Read the model definition and answer for the solid it produces. Units are mm, in the model's axes. A direction names the side the tool comes from. Round coordinates to 2 decimals unless told otherwise and drop trailing zeros. Write each loop counter-clockwise with the first axis right and the second up, starting at its lowest first coordinate (ties: lowest second). Pieces come first, ordered by that corner, then holes. Notation, with made-up numbers: (35.25, -14) - (61.25, -14) arc R16 cw to (61.25, 15) - close; hole circle Ø3 at (-33, 4.5). An arc over 180 degrees is marked (long way). One line per item, written item: value. Start each with the question number.
(1) A cutting plane is placed at D-D, the plane z = 36. Determine the outline of the cut face in (x, y), plus the area to 3 significant figures.
(2) Flat-ended cylindrical pins translate along their axes: pin 1 Ø2 at (x, y) = (7, -5) entering from -Z; pin 2 Ø3.5 at (x, z) = (15, 26) entering from -Y; pin 3 Ø8 at (x, z) = (22.5, 16) entering from -Y. Find the tip coordinate at first contact, or state that the pin passes through.
(3) A cutting plane is placed at A-A, the plane y = -12.25. Determine the outline of the cut face in (x, z), plus the area to 3 significant figures.
(4) The mould has two halves that part along X. Classify faces 1 (the face through (15, 0, 20)), 2 (the face through (12.34, -7.29, 12.68)), 3 (the face through (0, -9, 20)): +X half, -X half, draft (parallel to the pull), parting line (faces both ways), or undercut.
(5) A cutting plane is placed at C-C, the plane x = 3. Determine the outline of the cut face in (y, z), plus the area to 3 significant figures.
(6) A cutting plane is placed at B-B, the plane z = 31. Determine the outline of the cut face in (x, y), plus the area to 3 significant figures.
(7) For faces 4 (the face through (19.988, -13.435, 0.986)), 5 (the face through (15, -7, 40)), 6 (the face through (21.338, -0.435, 12.208)), 7 (the face through (15, -10, 20)), 8 (the face through (30, -9, 20)), determine the directions among +Z, -Z, +X, -X, +Y, -Y from which every point of the face is accessible in a straight line to the end or side of a thin tool.
(8) Find the intervals of material crossed by L1, parallel to X at y = -11, z = 16; L2, parallel to Z at x = 25.25, y = -12; L3, parallel to X at y = -7.25, z = 4, in increasing order.
from build123d import *

# Parameters (mm, degrees)
SKETCH_1_W          = 30
SKETCH_1_H          = 14
EXTRUDE_1_DEPTH     = 40
CUT_EXTRUDE_1_DEPTH = 35
SKETCH_4_W          = 27
SKETCH_4_H          = 36
CUT_EXTRUDE_2_DEPTH = 7.21308
SKETCH_5_R          = 0.565
CUT_EXTRUDE_3_DEPTH = 10
EXTRUDE_2_REACH     = 53.923
SKETCH_6_R          = 0.565
CUT_EXTRUDE_4_DEPTH = 1
SKETCH_8_R          = 0.565
CUT_EXTRUDE_5_DEPTH = 51.1269475


with BuildPart() as part:
    # 草图1 → 凸台-拉伸1 (new body)
    with BuildSketch(Plane.XY):
        with Locations((15, -7)):
            Rectangle(SKETCH_1_W, SKETCH_1_H)
    extrude(amount=EXTRUDE_1_DEPTH)

    # 草图3 → 切除-拉伸1 (cut)
    with BuildSketch(Plane(origin=(0, 0, 0), x_dir=(-1, 0, 0), z_dir=(0, 0, -1))):
        Polygon((-30, -4.5), (-25.764705882, -11.286920048), (-18.553603331, -6.786920048), (-22.788897449, 0), (-30, 0), align=None)
        Polygon((-7.211102551, 0), (-11.446396669, -6.786920048), (-4.235294118, -11.286920048), (0, -4.5), (0, 0), align=None)
    extrude(amount=-CUT_EXTRUDE_1_DEPTH, mode=Mode.SUBTRACT)

    # 草图4 → 切除-拉伸2 (cut)
    with BuildSketch(Plane.XZ.offset(14)):
        with Locations((15, 20)):
            Rectangle(SKETCH_4_W, SKETCH_4_H)
    extrude(amount=-CUT_EXTRUDE_2_DEPTH, mode=Mode.SUBTRACT)

    # 草图5 → 切除-拉伸3 (cut)
    with BuildSketch(Plane(origin=(0, 0, 0), x_dir=(-1, 0, 0), z_dir=(0, 0, -1))):
        with Locations((-10, -14)):
            Circle(SKETCH_5_R)
        with Locations((-20, -14)):
            Circle(SKETCH_5_R)
    extrude(amount=-CUT_EXTRUDE_3_DEPTH, mode=Mode.SUBTRACT)

    # 草图7 → 凸台-拉伸2 (add, up to next)
    with BuildSketch(Plane(origin=(0, 0, 0), x_dir=(-1, 0, 0), z_dir=(0, 0, -1)), mode=Mode.PRIVATE) as extrude_2_sk1:
        Polygon((-22.788897449, 0), (-18.553603331, -6.786920048), (-16.548520242, -10), (-13.451479758, -10), (-11.446396669, -6.786920048), (-7.211102551, 0), align=None)
    extrude_2_tool1 = extrude(extrude_2_sk1.sketch, amount=-EXTRUDE_2_REACH, mode=Mode.PRIVATE) - part.part
    add(extrude_2_tool1.solids().sort_by_distance((15, -3.886134, 0))[0])

    # 草图6 → 切除-拉伸4 (cut)
    with BuildSketch(Plane(origin=(5.189997684, 3.238754325, 0), x_dir=(0, 0, 1), z_dir=(-0.8483650059915271, -0.5294117647058821, 0))):
        with Locations(Location((12.2, -12.417642527, 0), (0, 0, 270))):
            Circle(SKETCH_6_R)
        with Locations(Location((12.2, -4.917642527, 0), (0, 0, 270))):
            Circle(SKETCH_6_R)
        with Locations(Location((4.2, -4.917642527, 0), (0, 0, 270))):
            Circle(SKETCH_6_R)
        with Locations(Location((19.97, -4.917642527, 0), (0, 0, 270))):
            Circle(SKETCH_6_R)
        with Locations(Location((27.74, -4.917642527, 0), (0, 0, 270))):
            Circle(SKETCH_6_R)
    cut_extrude_4 = extrude(amount=-CUT_EXTRUDE_4_DEPTH, mode=Mode.SUBTRACT)

    # 镜向1: 切除-拉伸4 across plane
    add(cut_extrude_4.mirror(Plane(origin=(15, 0, 0), x_dir=(0, 0, 1), z_dir=(1, 0, 0))), mode=Mode.SUBTRACT)

    # 草图8 → 切除-拉伸5 (cut, through all)
    with BuildSketch(Plane(origin=(5.189997684, 3.238754325, 0), x_dir=(0, 0, 1), z_dir=(-0.8483650059915271, -0.5294117647058821, 0))):
        with Locations(Location((12.2, -12.417642527, 0), (0, 0, 270))):
            Circle(SKETCH_8_R)
        with Locations(Location((4.2, -4.917642527, 0), (0, 0, 270))):
            Circle(SKETCH_8_R)
        with Locations(Location((27.74, -4.917642527, 0), (0, 0, 270))):
            Circle(SKETCH_8_R)
        with Locations(Location((19.97, -4.917642527, 0), (0, 0, 270))):
            Circle(SKETCH_8_R)
        with Locations(Location((12.2, -4.917642527, 0), (0, 0, 270))):
            Circle(SKETCH_8_R)
    extrude(amount=CUT_EXTRUDE_5_DEPTH, mode=Mode.SUBTRACT)


solid = part.part
Here are the results:
1. outline: (0, -14) - (1.5, -14) - (1.5, -6.79) - (11.45, -6.79) - (13.45, -10) - (16.55, -10) - (18.55, -6.79) - (28.5, -6.79) - (28.5, -14) - (30, -14) - (30, 0) - (0, 0) - close
1. area: 242 mm²
2. pin 1: z = 35
2. pin 2: y = -10
2. pin 3: y = -6.87
3. outline: (0, 0) - (30, 0) - (30, 40) - (0, 40) - close; hole (1.5, 2) - (28.5, 2) - (28.5, 38) - (1.5, 38) - close
3. area: 228 mm²
4. face 1: draft
4. face 2: undercut
4. face 3: -X half
5. outline: (-14, 0) - (-9.31, 0) - (-9.31, 2) - (-14, 2) - close; (-14, 38) - (-6.79, 38) - (-6.79, 35) - (0, 35) - (0, 40) - (-14, 40) - close
5. area: 57.7 mm²
6. outline: (0, -14) - (1.5, -14) - (1.5, -6.9) - (0, -4.5) - close; (7.21, 0) - (13.45, -10) - (16.55, -10) - (22.79, 0) - close; (28.5, -14) - (30, -14) - (30, -4.5) - (28.5, -6.9) - close
6. area: 118 mm²
7. face 4: -Z, -Y
7. face 5: +Z, +X, -X, +Y, -Y
7. face 6: none
7. face 7: -Y
7. face 8: +Z, -Z, +X, +Y, -Y
8. L1: 0 to 1.5, 28.5 to 30
8. L2: 0 to 2, 38 to 40
8. L3: 0 to 1.5, 11.74 to 18.26, 28.5 to 30
